from build123d import *

# Parameters (mm, degrees)
BASE_BRIDE_DEPTH          = 32
CONG_BRIDE1_R             = 0.5
ESQUISSE_ENL_V_MAT_BRID_W = 29
ESQUISSE_ENL_V_MAT_BRID_H = 12
ENL_V_MATI_RE_BRIDE_DEPTH = 59.216493896
CONG_BRIDE2_R             = 0.5
ESQUISSE_PERCAGE_BRIDE_R  = 5
PERCAGE_BRIDE_DEPTH       = 56.580213759
CHANFREIN_BRIDE_SIZE      = 0.2


with BuildPart() as part:
    # esquisse_base_bride → Base_bride (new body)
    with BuildSketch(Plane.XY):
        Polygon((40, 10), (44.330127019, 7.5), (44.330127019, -7.5), (40, -10), (-40, -10), (-40, 10), align=None)
    extrude(amount=BASE_BRIDE_DEPTH)

    # congé_bride1
    cong_bride1_edges = [part.edges().sort_by_distance(p)[0] for p in [
        (42.165063509, -8.75, 32),
        (-40, 10, 16),
        (44.330127019, 7.5, 16),
        (44.330127019, -7.5, 16),
        (-40, -10, 16),
        (44.330127019, 0, 32),
        (42.165063509, 8.75, 32),
        (0, 10, 32),
        (-40, 0, 32),
        (0, 10, 0),
        (42.165063509, 8.75, 0),
        (44.330127019, 0, 0),
        (0, -10, 32),
        (42.165063509, -8.75, 0),
        (0, -10, 0),
        (-40, 0, 0),
    ]]
    fillet(cong_bride1_edges, radius=CONG_BRIDE1_R)

    # esquisse_enlèv.mat.brid → enlèv.matière_bride (cut, through all)
    with BuildSketch(Plane(origin=(0, 10, 0), x_dir=(1, 0, 0), z_dir=(0, 1, 0))):
        with Locations((-25.5, -16)):
            Rectangle(ESQUISSE_ENL_V_MAT_BRID_W, ESQUISSE_ENL_V_MAT_BRID_H)
        with BuildLine():
            Line((4, -10.5), (24, -10.5))
            ThreePointArc((24, -10.5), (29.5, -16), (24, -21.5))
            Line((24, -21.5), (4, -21.5))
            ThreePointArc((4, -21.5), (-1.5, -16), (4, -10.5))
        make_face()
    extrude(amount=-ENL_V_MATI_RE_BRIDE_DEPTH, mode=Mode.SUBTRACT)

    # congé_bride2
    # the kernel refuses this fillet: 0.5 mm, written as the material it takes off along each edge
    with BuildSketch(Plane(origin=(-40.75, -10, 22), x_dir=(0, 1, 0), z_dir=(1, 0, 0))) as cong_bride2_piece_1:
        with BuildLine():
            CenterArc((CONG_BRIDE2_R, CONG_BRIDE2_R), CONG_BRIDE2_R, 180, 90)
            Line((0, CONG_BRIDE2_R), (0, 0))
            Line((0, 0), (CONG_BRIDE2_R, 0))
        make_face()
    extrude(amount=29.75, mode=Mode.SUBTRACT)
    with BuildSketch(Plane(origin=(-11, 10, 22), x_dir=(0, 0, 1), z_dir=(-1, 0, 0))) as cong_bride2_piece_2:
        with BuildLine():
            CenterArc((CONG_BRIDE2_R, -CONG_BRIDE2_R), CONG_BRIDE2_R, 90, 90)
            Line((0, -CONG_BRIDE2_R), (0, 0))
            Line((0, 0), (CONG_BRIDE2_R, 0))
        make_face()
    extrude(amount=29.75, mode=Mode.SUBTRACT)
    with BuildSketch(Plane(origin=(24, 10, 16), x_dir=(0, 0, -1), z_dir=(-1, 0, 0))) as cong_bride2_piece_3:
        with BuildLine():
            CenterArc((5.5 + CONG_BRIDE2_R, CONG_BRIDE2_R), CONG_BRIDE2_R, 180, 90)
            Line((5.5, CONG_BRIDE2_R), (5.5, 0))
            Line((5.5, 0), (5.5 + CONG_BRIDE2_R, 0))
        make_face()
    revolve(axis=Axis((24, 10, 16), (0, -1, 0)), revolution_arc=180, mode=Mode.SUBTRACT)
    with BuildSketch(Plane(origin=(4, 10, 10.5), x_dir=(0, 0, -1), z_dir=(1, 0, 0)), Plane(origin=(24, 10, 21.5), x_dir=(0, 0, 1), z_dir=(-1, 0, 0))) as cong_bride2_piece_4:
        with BuildLine():
            CenterArc((CONG_BRIDE2_R, -CONG_BRIDE2_R), CONG_BRIDE2_R, 90, 90)
            Line((0, -CONG_BRIDE2_R), (0, 0))
            Line((0, 0), (CONG_BRIDE2_R, 0))
        make_face()
    extrude(amount=20, mode=Mode.SUBTRACT)
    with BuildSketch(Plane(origin=(4, 10, 16), x_dir=(0, 0, 1), z_dir=(1, 0, 0))) as cong_bride2_piece_5:
        with BuildLine():
            CenterArc((5.5 + CONG_BRIDE2_R, CONG_BRIDE2_R), CONG_BRIDE2_R, 180, 90)
            Line((5.5, CONG_BRIDE2_R), (5.5, 0))
            Line((5.5, 0), (5.5 + CONG_BRIDE2_R, 0))
        make_face()
    revolve(axis=Axis((4, 10, 16), (0, -1, 0)), revolution_arc=180, mode=Mode.SUBTRACT)
    with BuildSketch(Plane(origin=(24, -10, 16), x_dir=(0, 0, 1), z_dir=(-1, 0, 0))) as cong_bride2_piece_6:
        with BuildLine():
            CenterArc((5.5 + CONG_BRIDE2_R, CONG_BRIDE2_R), CONG_BRIDE2_R, 180, 90)
            Line((5.5 + CONG_BRIDE2_R, 0), (5.5, 0))
            Line((5.5, 0), (5.5, CONG_BRIDE2_R))
        make_face()
    revolve(axis=Axis((24, -10, 16), (0, 1, 0)), revolution_arc=180, mode=Mode.SUBTRACT)
    with BuildSketch(Plane(origin=(24, -10, 10.5), x_dir=(0, 1, 0), z_dir=(-1, 0, 0)), Plane(origin=(4, -10, 21.5), x_dir=(0, 1, 0), z_dir=(1, 0, 0))) as cong_bride2_piece_7:
        with BuildLine():
            CenterArc((CONG_BRIDE2_R, CONG_BRIDE2_R), CONG_BRIDE2_R, 180, 90)
            Line((0, CONG_BRIDE2_R), (0, 0))
            Line((0, 0), (CONG_BRIDE2_R, 0))
        make_face()
    extrude(amount=20, mode=Mode.SUBTRACT)
    with BuildSketch(Plane(origin=(4, -10, 16), x_dir=(0, 0, -1), z_dir=(1, 0, 0))) as cong_bride2_piece_8:
        with BuildLine():
            CenterArc((5.5 + CONG_BRIDE2_R, CONG_BRIDE2_R), CONG_BRIDE2_R, 180, 90)
            Line((5.5 + CONG_BRIDE2_R, 0), (5.5, 0))
            Line((5.5, 0), (5.5, CONG_BRIDE2_R))
        make_face()
    revolve(axis=Axis((4, -10, 16), (0, 1, 0)), revolution_arc=180, mode=Mode.SUBTRACT)

    # esquisse_percage_bride → percage_bride (cut, through all)
    with BuildSketch(Plane.XY.offset(32)):
        with Locations((-30, 0)):
            Circle(ESQUISSE_PERCAGE_BRIDE_R)
    extrude(amount=-PERCAGE_BRIDE_DEPTH, mode=Mode.SUBTRACT)

    # chanfrein_bride
    chanfrein_bride_edges = [part.edges().sort_by_distance(p)[0] for p in [
        (-35, 0, 0),
        (-35, 0, 22),
        (-35, 0, 32),
    ]]
    chamfer(chanfrein_bride_edges, length=CHANFREIN_BRIDE_SIZE)


solid = part.part
Verification items for the finished model (mm, model axes). A direction names the side the tool comes from. Round coordinates to 2 decimals unless told otherwise and drop trailing zeros. Order: outer loops, then holes, each group sorted by start corner. A loop starts at its lowest first (then second) coordinate and runs counter-clockwise, first axis right, second up.
1. Release check for a two-part mould opening along X. For faces 4 (the cylindrical face through (-35, 0, 5)), 5 (the cylindrical face through (41.94, -8.715, 0.15)), 6 (the flat face through (-40, 0, 27)) record: +X half, -X half, draft (parallel to the pull), parting line (faces both ways), or undercut.
Final values:
face 4: undercut
face 5: +X half
face 6: -X half
2. Section check C-C on y = 0. State how many separate pieces and enclosed holes the cut face has, then the cut area to 3 significant figures.
Final values:
separate pieces: 3
enclosed holes: 1
area: 1,840 mm2
3. Access from +Z, -Z, +X, -X, +Y, -Y to the whole of each face (thin tool, end or side, straight path). Record for faces 1 (the flat face through (14, 0, 21.5)), 2 (the cylindrical face through (42, 8.68, 0.15)), 3 (the flat face through (-22, 0, 22)).
Final values:
face 1: +Y, -Y
face 2: -Z, +X, +Y
face 3: -X, +Y, -Y
4. Thickness scan on L1, parallel to Y at x = -30, z = 26; L2, parallel to Z at x = 7.5, y = -5.25; L3, parallel to Z at x = -36, y = 0.5. Record the ranges inside material, lowest first.
Final values:
L1: y = -10 to -5, 5 to 10
L2: z = 0 to 10.5, 21.5 to 32
L3: z = 0 to 10, 22 to 32
5. Section check A-A on z = 26. Record the cut outline in (x, y), then the cut area to 3 significant figures.
Final values:
outline: (-40, -9.5) arc R0.5 ccw to (-39.5, -10) - (40, -10) - (44.08, -7.64) arc R0.5 ccw to (44.33, -7.21) - (44.33, 7.21) arc R0.5 ccw to (44.08, 7.64) - (40, 10) - (-39.5, 10) arc R0.5 ccw to (-40, 9.5) - close; hole circle Ø10 at (-30, 0)
area: 1,600 mm2
6. Section check B-B on x = 18.5. Record the cut outline in (y, z).
Final values:
outline: (-10, 0.5) arc R0.5 ccw to (-9.5, 0) - (9.5, 0) arc R0.5 ccw to (10, 0.5) - (10, 10) arc R0.5 ccw to (9.5, 10.5) - (-9.5, 10.5) arc R0.5 ccw to (-10, 10) - close; (-10, 22) arc R0.5 ccw to (-9.5, 21.5) - (9.5, 21.5) arc R0.5 ccw to (10, 22) - (10, 31.5) arc R0.5 ccw to (9.5, 32) - (-9.5, 32) arc R0.5 ccw to (-10, 31.5) - close
7. Section check D-D on z = 16. Record the cut outline in (x, y).
Final values:
outline: (-11, -10) - (-2, -10) arc R0.5 ccw to (-1.5, -9.5) - (-1.5, 9.5) arc R0.5 ccw to (-2, 10) - (-11, 10) - close; (29.5, -9.5) arc R0.5 ccw to (30, -10) - (40, -10) - (44.08, -7.64) arc R0.5 ccw to (44.33, -7.21) - (44.33, 7.21) arc R0.5 ccw to (44.08, 7.64) - (40, 10) - (30, 10) arc R0.5 ccw to (29.5, 9.5) - close
